Geometry check sheet. Reference: the model listing, model coordinates, mm. A direction names the side the tool comes from. Coordinates: 2 decimals unless noted, no trailing zeros. Loops run counter-clockwise (first coordinate to the right, second up) from the corner with the lowest first, then second, coordinate; pieces in that order, holes last.
from build123d import *

# Parameters (mm, degrees)
MODEL_R             = 1.5
BOSS_EXTRUDE1_DEPTH = 2.8


with BuildPart() as part:
    # Model → Boss-Extrude1 (new body)
    with BuildSketch(Plane.XY):
        with BuildLine():
            Line((91.882047895, -12.427518263), (111.882047895, -12.427518263))
            Line((111.882047895, -12.427518263), (111.882047895, -2.427518263))
            Line((111.882047895, -2.427518263), (111.882047895, 12.572481737))
            ThreePointArc((111.882047895, 12.572481737), (110.417581801, 16.108015643), (106.882047895, 17.572481737))
            Line((106.882047895, 17.572481737), (96.882047895, 17.572481737))
            ThreePointArc((96.882047895, 17.572481737), (93.346513989, 16.108015643), (91.882047895, 12.572481737))
            Line((91.882047895, 12.572481737), (91.882047895, -2.427518263))
            Line((91.882047895, -2.427518263), (91.882047895, -12.427518263))
        make_face()
        with Locations((101.727306447, -7.427518263)):
            Circle(MODEL_R, mode=Mode.SUBTRACT)
        Polygon((101.882047895, 12.572481737), (96.882047895, 12.572481737), (96.882047895, 9.772481737), (106.882047895, 9.772481737), (106.882047895, 12.572481737), align=None, mode=Mode.SUBTRACT)
    extrude(amount=BOSS_EXTRUDE1_DEPTH)


solid = part.part
(1) Gauge pin test, flat end, axial feed: pin 1 Ø1 at (x, y) = (98, -5.5) entering from -Z. Record the tip position at first contact, or that the pin passes through.
Findings:
pin 1: stops at z = 0
(2) Scan lines: L1, parallel to Y at x = 99.5, z = 0.25; L2, parallel to Y at x = 102.75, z = 1.85; L3, parallel to X at y = 11.25, z = 1.15. Record each from-to range of solid material in increasing order.
Findings:
L1: y = -12.43 to 9.77, 12.57 to 17.57
L2: y = -12.43 to -8.52, -6.33 to 9.77, 12.57 to 17.57
L3: x = 91.88 to 96.88, 106.88 to 111.88
(3) Sectioned sample at A-A on x = 104. Record the cut outline in (y, z), and give its area (3 significant figures).
Findings:
outline: (-12.43, 0) - (9.77, 0) - (9.77, 2.8) - (-12.43, 2.8) - close; (12.57, 0) - (17.57, 0) - (17.57, 2.8) - (12.57, 2.8) - close
area: 76.2 mm2
(4) Sectioned sample at B-B on y = 12. Record the cut outline in (x, z), and give its area (3 significant figures).
Findings:
outline: (91.88, 0) - (96.88, 0) - (96.88, 2.8) - (91.88, 2.8) - close; (106.88, 0) - (111.88, 0) - (111.88, 2.8) - (106.88, 2.8) - close
area: 28.0 mm2
(5) Access from +Z, -Z, +X, -X, +Y, -Y to the whole of each face (thin tool, end or side, straight path). Record for faces 1 (the cylindrical face through (93.39, 16.15, 1.38)), 2 (the flat face through (102, 9.772, 1)).
Findings:
face 1: +Z, -Z, -X, +Y
face 2: +Z, -Z
(6) Sectioned sample at C-C on z = 0.9. Record the cut outline in (x, y), and give its area (3 significant figures).
Findings:
outline: (91.88, -12.43) - (111.88, -12.43) - (111.88, 12.57) arc R5 ccw to (106.88, 17.57) - (96.88, 17.57) arc R5 ccw to (91.88, 12.57) - close; hole (96.88, 9.77) - (106.88, 9.77) - (106.88, 12.57) - (96.88, 12.57) - close; hole circle Ø3 at (101.73, -7.43)
area: 554 mm2
(7) Sectioned sample at D-D on x = 109.75. Record the cut outline in (y, z).
Findings:
outline: (-12.43, 0) - (16.67, 0) - (16.67, 2.8) - (-12.43, 2.8) - close
(8) Draft check along Y on faces 3 (the flat face through (111.882, 0, 1)), 4 (the cylindrical face through (110.456, 16.069, 1.38)), 5 (the flat face through (106.882, 11, 1)), 6 (the flat face through (102, -12.428, 1)). Enter one of: +Y half, -Y half, draft (parallel to the pull), parting line (faces both ways), or undercut.
Findings:
face 3: draft
face 4: +Y half
face 5: undercut
face 6: -Y half
